Part model, mm, in its own coordinate system. A direction names the side the tool comes from. Coordinates: 2 decimals unless noted, no trailing zeros. Order: outer loops, then holes, each group sorted by start corner. A loop starts at its lowest first (then second) coordinate and runs counter-clockwise, first axis right, second up. Notation, with made-up numbers: M -39,-12.75 L -27,-12.75 A28 cw -27,15.25 Z; hole C 67,-14 d2. An arc over 180 degrees is marked long. Write item = value, one per line. Start each with the question number.
from build123d import *

# Parameters (mm, degrees)
BOSS_EXTRUDE1_DEPTH                            = 20
SKETCH2_R                                      = 1.27
CUT_EXTRUDE1_DEPTH                             = 4.000000128
SKETCH3_R                                      = 4.8006
CUT_EXTRUDE2_DEPTH                             = 3.175
SKETCH4_R                                      = 3.81
CUT_EXTRUDE3_DEPTH                             = 0.254
CUT_EXTRUDE4_START                             = -3.175
SKETCH5_R                                      = 4.8006
CUT_EXTRUDE4_DEPTH                             = 3.175
CUT_EXTRUDE5_START                             = -0.254
SKETCH6_R                                      = 3.81
CUT_EXTRUDE5_DEPTH                             = 0.254
CBORE_FOR_0_SOCKET_HEAD_CAP_SCREW1_D           = 1.778
CBORE_FOR_0_SOCKET_HEAD_CAP_SCREW1_CBORE_D     = 3.175
CBORE_FOR_0_SOCKET_HEAD_CAP_SCREW1_CBORE_DEPTH = 14.732
FILLET1_R                                      = 2.54


with BuildPart() as part:
    # Sketch1 → Boss-Extrude1 (new body)
    with BuildSketch(Plane.XY):
        Polygon((-71.742285041, 0), (-71.742285041, -4), (-53.530479711, -4), (-53.530479711, 11.43), (-61.150490131, 11.43), (-61.150490131, 0), align=None)
    extrude(amount=-BOSS_EXTRUDE1_DEPTH)

    # Sketch2 → Cut-Extrude1 (cut)
    with BuildSketch(Plane.ZY.offset(71.742285041)):
        with Locations((-12.286, -2)):
            Circle(SKETCH2_R)
        with Locations(Location((-7.714, -2, 0), (0, 0, 180))):
            Circle(SKETCH2_R)
    extrude(amount=-CUT_EXTRUDE1_DEPTH, mode=Mode.SUBTRACT)

    # Sketch3 → Cut-Extrude2 (cut)
    with BuildSketch(Plane.ZY.offset(61.150490131)):
        with Locations((-10, 5.08)):
            Circle(SKETCH3_R)
    extrude(amount=-CUT_EXTRUDE2_DEPTH, mode=Mode.SUBTRACT)

    # Sketch4 → Cut-Extrude3 (cut)
    with BuildSketch(Plane.ZY.offset(57.975490131)):
        with Locations((-10, 5.08)):
            Circle(SKETCH4_R)
    extrude(amount=-CUT_EXTRUDE3_DEPTH, mode=Mode.SUBTRACT)

    # Sketch5 → Cut-Extrude4 (cut)
    with BuildSketch(Plane(origin=(-53.530479711, 0, 0), x_dir=(0, 0, -1), z_dir=(1, 0, 0)).offset(CUT_EXTRUDE4_START)):
        with Locations(Location((10, 5.08, 0), (0, 0, 180))):
            Circle(SKETCH5_R)
    extrude(amount=CUT_EXTRUDE4_DEPTH, mode=Mode.SUBTRACT)

    # Sketch6 → Cut-Extrude5 (cut)
    with BuildSketch(Plane(origin=(-56.705479711, 0, 0), x_dir=(0, 0, -1), z_dir=(1, 0, 0)).offset(CUT_EXTRUDE5_START)):
        with Locations(Location((10, 5.08, 0), (0, 0, 180))):
            Circle(SKETCH6_R)
    extrude(amount=CUT_EXTRUDE5_DEPTH, mode=Mode.SUBTRACT)

    # CBORE for #0 Socket Head Cap Screw1 (through all)
    with Locations(Plane.ZY.offset(71.742285041)):
        with Locations((-16.952, -2.032), (-3.048, -2.032)):
            CounterBoreHole(CBORE_FOR_0_SOCKET_HEAD_CAP_SCREW1_D / 2, CBORE_FOR_0_SOCKET_HEAD_CAP_SCREW1_CBORE_D / 2, CBORE_FOR_0_SOCKET_HEAD_CAP_SCREW1_CBORE_DEPTH)

    # Fillet1
    # the kernel refuses this fillet: 2.54 mm, written as the material it takes off along each edge
    with BuildSketch(Plane(origin=(-78.092285041, -4, -20), x_dir=(0, 1, 0), z_dir=(1, 0, 0))) as fillet1_piece_1:
        with BuildLine():
            CenterArc((FILLET1_R, FILLET1_R), FILLET1_R, 180, 90)
            Line((0, FILLET1_R), (0, 0))
            Line((0, 0), (FILLET1_R, 0))
        make_face()
    extrude(amount=30.91180533, mode=Mode.SUBTRACT)
    with BuildSketch(Plane(origin=(-61.150490131, 11.43, 6.35), x_dir=(0, -1, 0), z_dir=(0, 0, -1))) as fillet1_piece_2:
        with BuildLine():
            CenterArc((FILLET1_R, -FILLET1_R), FILLET1_R, 90, 90)
            Line((0, -FILLET1_R), (0, 0))
            Line((0, 0), (FILLET1_R, 0))
        make_face()
    extrude(amount=32.7, mode=Mode.SUBTRACT)
    with BuildSketch(Plane(origin=(-61.150490131, 17.78, -20), x_dir=(1, 0, 0), z_dir=(0, -1, 0))) as fillet1_piece_3:
        with BuildLine():
            CenterArc((FILLET1_R, FILLET1_R), FILLET1_R, 180, 90)
            Line((0, FILLET1_R), (0, 0))
            Line((0, 0), (FILLET1_R, 0))
        make_face()
    extrude(amount=17.78, mode=Mode.SUBTRACT)
    with BuildSketch(Plane(origin=(-61.150490131, 17.78, 0), x_dir=(1, 0, 0), z_dir=(0, -1, 0))) as fillet1_piece_4:
        with BuildLine():
            CenterArc((FILLET1_R, -FILLET1_R), FILLET1_R, 90, 90)
            Line((0, -FILLET1_R), (0, 0))
            Line((0, 0), (FILLET1_R, 0))
        make_face()
    extrude(amount=17.78, mode=Mode.SUBTRACT)
    with BuildSketch(Plane(origin=(-78.092285041, -4, 0), x_dir=(0, 1, 0), z_dir=(1, 0, 0))) as fillet1_piece_5:
        with BuildLine():
            CenterArc((FILLET1_R, -FILLET1_R), FILLET1_R, 90, 90)
            Line((0, -FILLET1_R), (0, 0))
            Line((0, 0), (FILLET1_R, 0))
        make_face()
    extrude(amount=30.91180533, mode=Mode.SUBTRACT)


solid = part.part
Item 1: Cut at D-D, the plane z = -14.25. Write the cut outline in (x, y).
Item 2: Flat gauge pins, fed straight in: pin 1 (5 mm diameter, centred on x = -62.5, z = -3, fed in from +Y); pin 2 (2.5 mm diameter, centred on y = 4, z = -10.5, fed in from -X); pin 3 (8.5 mm diameter, centred on y = 5.08, z = -10, fed in from +X); pin 4 (4 mm diameter, centred on y = -2.032, z = -16.952, fed in from +X). Where does each tip first touch, or does it go through?
Item 3: 3-axis set-ups, long thin cutter, end or side, ignore diameter. For faces 1 (the cylindrical face through (-60.387, 5.795, -0.724)), 2 (the cylindrical face through (-64.479, -1.555, -15.438)), 3 (the flat face through (-56.959, 5, -10)), 4 (the flat face through (-61.15, 5, -5)), 5 (the cylindrical face through (-60.426, 5.795, -19.236)): which of +Z, -Z, +X, -X, +Y, -Y reach the whole face in a straight line?
Item 4: Cut at A-A, the plane y = 5.08. Write the cut outline in (x, z).
Item 5: Wall check: line 1 along Y through (x, z) = (-55.75, -10.25); line 2 along Y through (x, z) = (-67.5, -8); line 3 along X through (y, z) = (7, -4.25). Give the ranges that are in metal, low to high. Write a range as [from, to].
Item 6: Cut at C-C, the plane x = -55.75. Write the cut outline in (y, z).
Item 7: Cut at B-B, the plane z = -3. Write the cut outline in (x, y).
Filled sheet:
q1.outline = M -71.74,-4 L -53.53,-4 L -53.53,2.85 L -56.71,2.85 L -56.71,7.31 L -53.53,7.31 L -53.53,11.43 L -58.61,11.43 A2.54 ccw -61.15,8.89 L -61.15,7.31 L -57.98,7.31 L -57.98,2.85 L -61.15,2.85 L -61.15,0 L -71.74,0 Z
q2.pin_1 = 11.02
q2.pin_2 = -57.72
q2.pin_3 = -56.71
q2.pin_4 = -53.53
q3.face_1 = +Z, -X, +Y
q3.face_2 = -X
q3.face_3 = +X
q3.face_4 = +Z, -Z, -X, +Y
q3.face_5 = -Z, -X, +Y
q4.outline = M -61.15,-17.46 A2.54 ccw -58.61,-20 L -53.53,-20 L -53.53,-14.8 L -56.71,-14.8 L -56.71,-13.81 L -56.96,-13.81 L -56.96,-6.19 L -56.71,-6.19 L -56.71,-5.2 L -53.53,-5.2 L -53.53,0 L -58.61,0 A2.54 ccw -61.15,-2.54 L -61.15,-5.2 L -57.98,-5.2 L -57.98,-6.19 L -57.72,-6.19 L -57.72,-13.81 L -57.98,-13.81 L -57.98,-14.8 L -61.15,-14.8 Z
q5.line_1 = [-4, 0.29], [9.87, 11.43]
q5.line_2 = [-4, 0]
q5.line_3 = [-61.15, -53.53]
q6.outline = M -4,-17.46 A2.54 ccw -1.46,-20 L 11.43,-20 L 11.43,0 L -1.46,0 A2.54 ccw -4,-2.54 Z; hole C -2.03,-16.95 d1.78; hole C -2.03,-3.05 d1.78; hole C 5.08,-10 d9.6
q7.outline = M -71.74,-4 L -53.53,-4 L -53.53,-2.92 L -57.01,-2.92 L -57.01,-3.62 L -71.74,-3.62 Z; M -71.74,-0.45 L -57.01,-0.45 L -57.01,-1.14 L -53.53,-1.14 L -53.53,11.43 L -58.61,11.43 A2.54 ccw -61.15,8.89 L -61.15,0 L -71.74,0 Z
